Check sheet for the drawn part. Datum: minimum x, y, z corner. Units: mm. Round coordinates to 2 decimals unless told otherwise and drop trailing zeros. Order: outer loops, then holes, each group sorted by start corner. A loop starts at its lowest first (then second) coordinate and runs counter-clockwise, first axis right, second up. Notation, with made-up numbers: (-31.75, 87.25) - (16.25, 87.25) arc R21 ccw to (16.25, 95.25) - close; hole circle Ø2 at (17.5, -10.5). An arc over 180 degrees is marked (long way). Write each question's results on one line, items separated by ' | '.
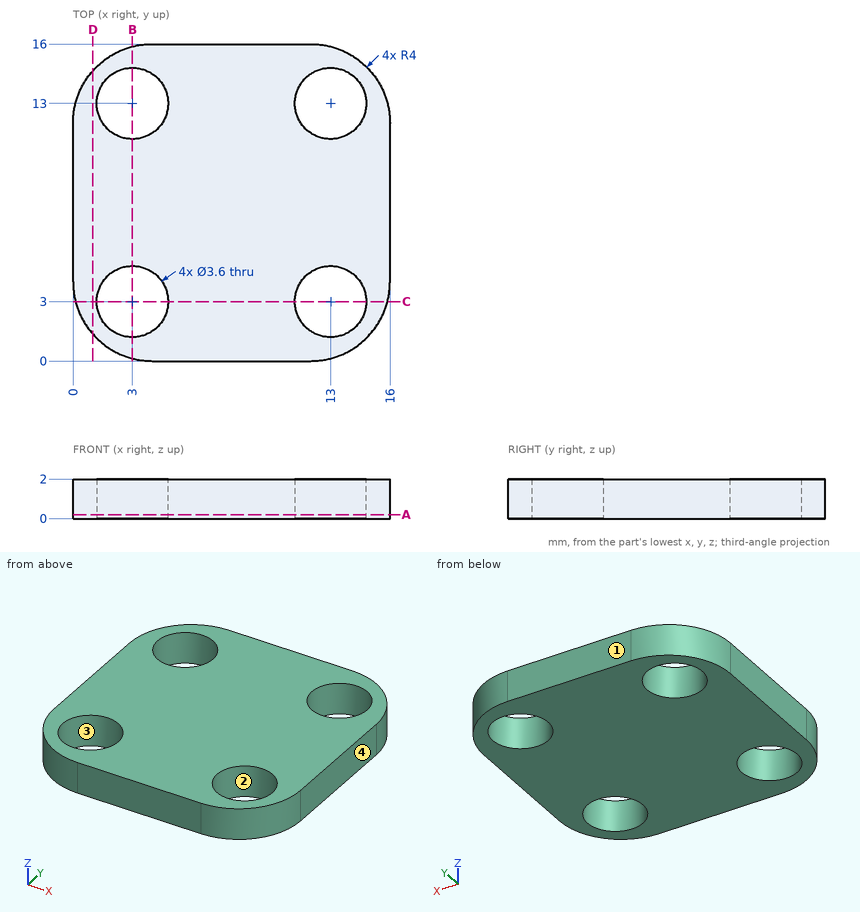
(1) Section check A-A (z = 0.2). Record the cut outline in (x, y).
Answers follow:
outline: (0, 4) arc R4 ccw to (4, 0) - (12, 0) arc R4 ccw to (16, 4) - (16, 12) arc R4 ccw to (12, 16) - (4, 16) arc R4 ccw to (0, 12) - close; hole circle Ø3.6 at (3, 3); hole circle Ø3.6 at (3, 13); hole circle Ø3.6 at (13, 3); hole circle Ø3.6 at (13, 13)
(2) Draft check along Y on the marked faces 1, 2, 3 and 4. Enter one of: released by +Y, released by -Y, zero draft, split by the parting line, or undercut.
Answers follow:
face 1: released by +Y | face 2: undercut | face 3: undercut | face 4: zero draft
(3) Section check D-D (x = 1). Record the cut outline in (y, z).
Answers follow:
outline: (1.35, 0) - (14.65, 0) - (14.65, 2) - (1.35, 2) - close
(4) Material ranges on line 1 (Y direction, x = 2.25, z = 1.1); line 2 (Y direction, x = 3, z = 0.4), recorded low to high.
Answers follow:
line 1: 0.4 to 1.36, 4.64 to 11.36, 14.64 to 15.6 | line 2: 0.13 to 1.2, 4.8 to 11.2, 14.8 to 15.87
(5) Section check B-B (x = 3). Record the cut outline in (y, z).
Answers follow:
outline: (0.13, 0) - (1.2, 0) - (1.2, 2) - (0.13, 2) - close; (4.8, 0) - (11.2, 0) - (11.2, 2) - (4.8, 2) - close; (14.8, 0) - (15.87, 0) - (15.87, 2) - (14.8, 2) - close
